```python
from build123d import *

# Parameters (mm, degrees)
BOSS_EXTRUDE1_DEPTH = 8
SKETCH5_W           = 1.5
SKETCH5_H           = 2.448371941
BOSS_EXTRUDE4_DEPTH = 2
SKETCH6_R           = 3
CUT_EXTRUDE1_DEPTH  = 265.555525233
FILLET1_R           = 4


with BuildPart() as part:
    # Sketch1 → Boss-Extrude1 (new body)
    with BuildSketch(Plane.XY):
        Polygon((-118.155372005, 57.283765903), (-198.155372005, 57.283765903), (-250.845489232, 41.511906575), (-258.155372005, 7.283765903), (-254.866788986, 7.283765903), (-248.926231582, 35.100112729), (-198.155372005, 47.283765903), (-118.155372005, 47.283765903), align=None)
    extrude(amount=BOSS_EXTRUDE1_DEPTH)

    # Sketch5 → Boss-Extrude4 (add)
    with BuildSketch(Plane.XZ.offset(-47.283765903)):
        Polygon((-128.155372005, 6.5), (-119.655372005, 6.5), (-118.155372005, 6.5), (-118.155372005, 8), (-128.155372005, 8), align=None)
        Polygon((-119.655372005, 4.051628059), (-119.655372005, 3.948371941), (-118.155372005, 3.948371941), (-118.155372005, 6.5), (-119.655372005, 6.5), align=None)
        with Locations((-118.905372005, 2.724185971)):
            Rectangle(SKETCH5_W, SKETCH5_H)
        Polygon((-118.155372005, 1.5), (-119.655372005, 1.5), (-128.155372005, 1.5), (-128.155372005, 0), (-118.155372005, 0), align=None)
    extrude(amount=BOSS_EXTRUDE4_DEPTH)

    # Sketch6 → Cut-Extrude1 (cut, through all)
    with BuildSketch(Plane.XY.offset(8)):
        with Locations((-194.405761522, 52.286388284)):
            Circle(SKETCH6_R)
    extrude(amount=-CUT_EXTRUDE1_DEPTH, mode=Mode.SUBTRACT)

    # Fillet1
    fillet1_edges = [part.edges().sort_by_distance(p)[0] for p in [
        (-248.926231582, 35.100112729, 4),
        (-250.845489232, 41.511906575, 4),
        (-256.511080495, 7.283765903, 0),
        (-256.511080495, 7.283765903, 8),
    ]]
    fillet(fillet1_edges, radius=FILLET1_R - 0.0001)  # a hair under: the kernel refuses the full size


solid = part.part
```
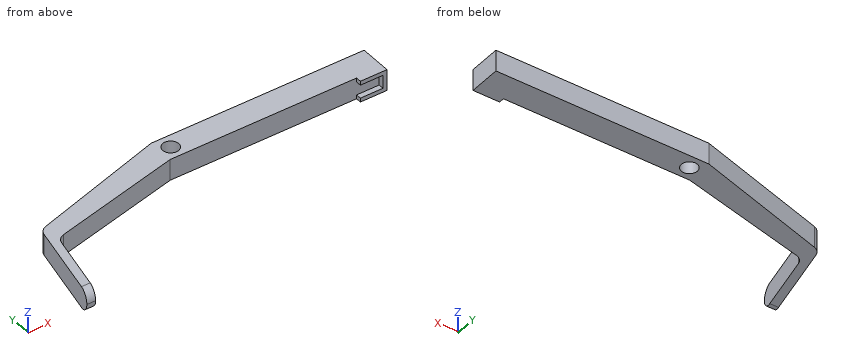
Part model, mm, in its own coordinate system. Give positions to 0.01 mm unless a question says otherwise; leave off trailing zeros. Write each loop counter-clockwise with the first axis right and the second up, starting at its lowest first coordinate (ties: lowest second). Pieces come first, ordered by that corner, then holes. Notation, with made-up numbers: (43, 1.25) -> (101, 1.25) arc R29 ccw to (101, 23.25) -> close; hole circle Ø10 at (2, -39). An arc over 180 degrees is marked (long way). Put each result on its own line as item: value. Start each with the question number.
Item 1: Cut at B-B (z = 5.25). List the corners of the cut face in (x, y).
Item 2: Wall check: L1, parallel to Y at x = -138.5, z = 2; L2, parallel to Z at x = -126, y = 46; L3, parallel to Y at x = -195, z = 1.5. Give the ranges that are in metal, low to high. Write a range as [from, to].
Item 3: Cut at D-D (y = 25). List the corners of the cut face in (x, z).
Item 4: Cut at C-C (x = -167). List the corners of the cut face in (y, z), then the cut area to 3 significant figures.
Item 5: Pin check, flat tips, straight feed: pin 1 Ø4 at (y, z) = (28.5, 2) entering from +X; pin 2 Ø5.5 at (x, y) = (-194.41, 52.29) entering from -Z; pin 3 Ø2 at (x, z) = (-180.5, 4) entering from -Y; pin 4 Ø2 at (y, z) = (39, 3) entering from -X. Stop position of each tip, or through.
Item 6: Cut at A-A (y = 53.5). List the corners of the cut face in (x, z), then the cut area to 3 significant figures.
Answer list:
1. outline: (-258.11, 7.48) -> (-254.82, 7.48) -> (-249.45, 32.63) arc R4 cw to (-246.47, 35.69) -> (-198.16, 47.28) -> (-119.66, 47.28) -> (-119.66, 45.28) -> (-118.16, 45.28) -> (-118.16, 57.28) -> (-198.16, 57.28) -> (-248.58, 42.19) arc R4 ccw to (-251.34, 39.19) -> close; hole circle Ø6 at (-194.41, 52.29)
2. L1: y = [47.28, 57.28]
2. L2: z = [0, 1.5], [6.5, 8]
2. L3: y = [47.28, 49.35], [55.23, 57.28]
3. outline: (-254.37, 0) -> (-251.08, 0) -> (-251.08, 8) -> (-254.37, 8) -> close
4. outline: (47.28, 0) -> (57.28, 0) -> (57.28, 8) -> (47.28, 8) -> close
4. area: 80.0 mm2
5. pin 1: stops at x = -249.91
5. pin 2: passes through
5. pin 3: stops at y = 47.28
5. pin 4: stops at x = -251.6
6. outline: (-210.8, 0) -> (-197.15, 0) -> (-197.15, 8) -> (-210.8, 8) -> close; (-191.66, 0) -> (-118.16, 0) -> (-118.16, 8) -> (-191.66, 8) -> close
6. area: 697 mm2
